from build123d import *

# Parameters (mm, degrees)
F0_R     = 4.665
F1_DEPTH = 6


with BuildPart() as f1:
    # F0 (on Front) → F1 (new body)
    with BuildSketch(Plane.XZ):
        with BuildLine():
            Line((186.500065, 187), (13.500065, 187))
            Line((13.500065, 187), (13.500065, 161.75))
            Line((13.500065, 161.75), (19.200065, 161.75))
            ThreePointArc((19.200065, 161.75), (19.412197, 161.837868), (19.500065, 162.05))
            Line((19.500065, 162.05), (19.500065, 162.8))
            ThreePointArc((19.500065, 162.8), (19.358643, 163.141421), (19.700065, 163))
            Line((19.700065, 163), (21.800065, 163))
            ThreePointArc((21.800065, 163), (22.141486, 163.141421), (22.000065, 162.8))
            Line((22.000065, 162.8), (22.000065, 162.05))
            ThreePointArc((22.000065, 162.05), (22.087933, 161.837868), (22.300065, 161.75))
            Line((22.300065, 161.75), (24.000065, 161.75))
            Line((24.000065, 161.75), (24.000065, 158.75))
            Line((24.000065, 158.75), (22.300065, 158.75))
            ThreePointArc((22.300065, 158.75), (22.087933, 158.662132), (22.000065, 158.45))
            Line((22.000065, 158.45), (22.000065, 157.7))
            ThreePointArc((22.000065, 157.7), (22.141486, 157.358579), (21.800065, 157.5))
            Line((21.800065, 157.5), (19.700065, 157.5))
            ThreePointArc((19.700065, 157.5), (19.358643, 157.358579), (19.500065, 157.7))
            Line((19.500065, 157.7), (19.500065, 158.45))
            ThreePointArc((19.500065, 158.45), (19.412197, 158.662132), (19.200065, 158.75))
            Line((19.200065, 158.75), (13.500065, 158.75))
            Line((13.500065, 158.75), (13.500065, 133.6))
            Line((13.500065, 133.6), (7.500065, 133.6))
            Line((7.500065, 133.6), (7.500065, 133.5))
            Line((7.500065, 133.5), (7.500065, 53.5))
            Line((7.500065, 53.5), (7.500065, 53.4))
            Line((7.500065, 53.4), (13.500109, 53.4))
            Line((13.500109, 53.4), (13.500072, 20.339))
            Line((13.500072, 20.339), (19.200072, 20.339))
            ThreePointArc((19.200072, 20.339), (19.412204, 20.426868), (19.500072, 20.639))
            Line((19.500072, 20.639), (19.500072, 21.389))
            ThreePointArc((19.500072, 21.389), (19.35865, 21.730421), (19.700072, 21.589))
            Line((19.700072, 21.589), (21.800072, 21.589))
            ThreePointArc((21.800072, 21.589), (22.141493, 21.730421), (22.000072, 21.389))
            Line((22.000072, 21.389), (22.000072, 20.639))
            ThreePointArc((22.000072, 20.639), (22.08794, 20.426868), (22.300072, 20.339))
            Line((22.300072, 20.339), (24.000068, 20.339))
            Line((24.000068, 20.339), (24.000068, 17.339))
            Line((24.000068, 17.339), (22.300068, 17.339))
            ThreePointArc((22.300068, 17.339), (22.087936, 17.251132), (22.000068, 17.039))
            Line((22.000068, 17.039), (22.000068, 16.289))
            ThreePointArc((22.000068, 16.289), (22.14149, 15.947579), (21.800068, 16.089))
            Line((21.800068, 16.089), (19.700068, 16.089))
            ThreePointArc((19.700068, 16.089), (19.358647, 15.947579), (19.500068, 16.289))
            Line((19.500068, 16.289), (19.500068, 17.039))
            ThreePointArc((19.500068, 17.039), (19.4122, 17.251132), (19.200068, 17.339))
            Line((19.200068, 17.339), (13.500068, 17.339))
            Line((13.500068, 17.339), (13.500031, -15.822))
            Line((13.500031, -15.822), (74.000065, -15.822))
            Line((74.000065, -15.822), (74.000065, 0))
            Line((74.000065, 0), (74.000065, 35))
            Line((74.000065, 35), (126.000065, 35))
            Line((126.000065, 35), (126.000065, 0))
            Line((126.000065, 0), (126.000065, -15.822))
            Line((126.000065, -15.822), (186.500098, -15.822))
            Line((186.500098, -15.822), (186.500061, 17.339))
            Line((186.500061, 17.339), (180.800061, 17.339))
            ThreePointArc((180.800061, 17.339), (180.587929, 17.251132), (180.500061, 17.039))
            Line((180.500061, 17.039), (180.500061, 16.289))
            ThreePointArc((180.500061, 16.289), (180.641482, 15.947579), (180.300061, 16.089))
            Line((180.300061, 16.089), (178.200058, 16.089))
            ThreePointArc((178.200058, 16.089), (177.858636, 15.947579), (178.000058, 16.289))
            Line((178.000058, 16.289), (178.000058, 17.039))
            ThreePointArc((178.000058, 17.039), (177.91219, 17.251132), (177.700058, 17.339))
            Line((177.700058, 17.339), (176.000058, 17.339))
            Line((176.000058, 17.339), (176.000058, 20.339))
            Line((176.000058, 20.339), (177.700058, 20.339))
            ThreePointArc((177.700058, 20.339), (177.91219, 20.426868), (178.000058, 20.639))
            Line((178.000058, 20.639), (178.000058, 21.389))
            ThreePointArc((178.000058, 21.389), (177.858636, 21.730421), (178.200058, 21.589))
            Line((178.200058, 21.589), (180.300058, 21.589))
            ThreePointArc((180.300058, 21.589), (180.641479, 21.730421), (180.500058, 21.389))
            Line((180.500058, 21.389), (180.500058, 20.639))
            ThreePointArc((180.500058, 20.639), (180.587926, 20.426868), (180.800058, 20.339))
            Line((180.800058, 20.339), (186.500058, 20.339))
            Line((186.500058, 20.339), (186.500021, 53.4))
            Line((186.500021, 53.4), (192.500065, 53.4))
            Line((192.500065, 53.4), (192.500065, 53.5))
            Line((192.500065, 53.5), (192.500065, 133.5))
            Line((192.500065, 133.5), (192.500065, 133.6))
            Line((192.500065, 133.6), (186.500065, 133.6))
            Line((186.500065, 133.6), (186.500065, 158.75))
            Line((186.500065, 158.75), (180.800058, 158.75))
            ThreePointArc((180.800058, 158.75), (180.587926, 158.662132), (180.500058, 158.45))
            Line((180.500058, 158.45), (180.500058, 157.7))
            ThreePointArc((180.500058, 157.7), (180.641479, 157.358579), (180.300058, 157.5))
            Line((180.300058, 157.5), (178.200058, 157.5))
            ThreePointArc((178.200058, 157.5), (177.858636, 157.358579), (178.000058, 157.7))
            Line((178.000058, 157.7), (178.000058, 158.45))
            ThreePointArc((178.000058, 158.45), (177.91219, 158.662132), (177.700058, 158.75))
            Line((177.700058, 158.75), (176.000058, 158.75))
            Line((176.000058, 158.75), (176.000058, 161.75))
            Line((176.000058, 161.75), (177.700058, 161.75))
            ThreePointArc((177.700058, 161.75), (177.91219, 161.837868), (178.000058, 162.05))
            Line((178.000058, 162.05), (178.000058, 162.8))
            ThreePointArc((178.000058, 162.8), (177.858636, 163.141421), (178.200058, 163))
            Line((178.200058, 163), (180.300065, 163))
            ThreePointArc((180.300065, 163), (180.641486, 163.141421), (180.500065, 162.8))
            Line((180.500065, 162.8), (180.500065, 162.05))
            ThreePointArc((180.500065, 162.05), (180.587933, 161.837868), (180.800065, 161.75))
            Line((180.800065, 161.75), (186.500065, 161.75))
            Line((186.500065, 161.75), (186.500065, 187))
        make_face()
        with BuildLine():
            Line((66.500065, -11.322), (66.500065, -8.322))
            ThreePointArc((66.500065, -8.322), (68.000065, -6.822), (69.500065, -8.322))
            Line((69.500065, -8.322), (69.500065, -11.322))
            ThreePointArc((69.500065, -11.322), (68.000065, -12.822), (66.500065, -11.322))
        make_face(mode=Mode.SUBTRACT)
        Polygon((28.62622, 48.081567), (28.837529, 48.534721), (65.08984, 31.629991), (64.878531, 31.176837), align=None, mode=Mode.SUBTRACT)
        with BuildLine():
            Line((130.500065, -11.322), (130.500065, -8.322))
            ThreePointArc((130.500065, -8.322), (132.000065, -6.822), (133.500065, -8.322))
            Line((133.500065, -8.322), (133.500065, -11.322))
            ThreePointArc((133.500065, -11.322), (132.000065, -12.822), (130.500065, -11.322))
        make_face(mode=Mode.SUBTRACT)
        with Locations((100.000065, 44.5)):
            Circle(F0_R, mode=Mode.SUBTRACT)
        Polygon((135.121598, 31.176837), (134.910289, 31.629991), (171.1626, 48.534721), (171.37391, 48.081567), align=None, mode=Mode.SUBTRACT)
        with BuildLine():
            ThreePointArc((9.000065, 93.75), (10.500065, 95.25), (12.000065, 93.75))
            Line((12.000065, 93.75), (12.000065, 93.25))
            ThreePointArc((12.000065, 93.25), (10.500065, 91.75), (9.000065, 93.25))
            Line((9.000065, 93.25), (9.000065, 93.75))
        make_face(mode=Mode.SUBTRACT)
        with BuildLine():
            Line((191.000064, 93.75), (191.000064, 93.25))
            ThreePointArc((191.000064, 93.25), (189.500064, 91.75), (188.000064, 93.25))
            Line((188.000064, 93.25), (188.000064, 93.75))
            ThreePointArc((188.000064, 93.75), (189.500064, 95.25), (191.000064, 93.75))
        make_face(mode=Mode.SUBTRACT)
    extrude(amount=F1_DEPTH)


solid = f1.part
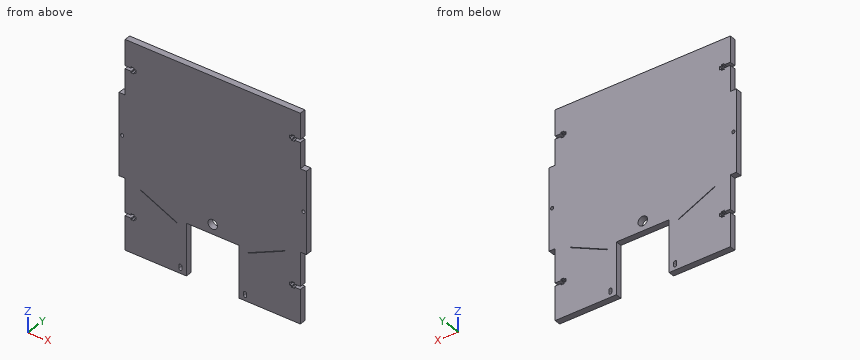
Work out the finished part from the listing and answer in its coordinate system (mm). Round coordinates to 2 decimals unless told otherwise and drop trailing zeros. Loops run counter-clockwise (first coordinate to the right, second up) from the corner with the lowest first, then second, coordinate; pieces in that order, holes last. Notation, with made-up numbers: (-9.75, 70.5) - (1.25, 70.5) arc R3 ccw to (1.25, 75.5) - close; hole circle Ø9 at (-7, -29). An arc over 180 degrees is marked (long way). One line per item, written item: value.
Q1. Find section A-A on z = 44.5. Give the vertices of the cut face in (x, y), and give its area (3 significant figures).
Check values:
outline: (13.5, -6) - (36.31, -6) - (36.31, 0) - (13.5, 0) - close; (37.49, -6) - (95.34, -6) - (95.34, 0) - (37.49, 0) - close; (104.67, -6) - (162.51, -6) - (162.51, 0) - (104.67, 0) - close; (163.69, -6) - (186.5, -6) - (186.5, 0) - (163.69, 0) - close
area: 968 mm2
Q2. Find section C-C on x = 107.5. Give the vertices of the cut face in (y, z).
Check values:
outline: (-6, 35) - (0, 35) - (0, 187) - (-6, 187) - close
Q3. Straight lines are drawn through the part: probe 1 along Z at (x, y) = (185, -5.7); probe 2 along X at (y, z) = (-3.6, 15.5); probe 3 along Z at (x, y) = (100, -2.9) (3 decimals). For each, find the intervals that lie inside material, in ascending order.
Check values:
probe 1: -15.82 to 17.34, 20.34 to 158.75, 161.75 to 187
probe 2: 13.5 to 74, 126 to 186.5
probe 3: 35 to 39.835, 49.165 to 187
Q4. Find section B-B on y = -2. State how many separate pieces and enclosed holes the cut face has, and give its area (3 significant figures).
Check values:
separate pieces: 1
enclosed holes: 7
area: 33,100 mm2
Q5. Each of these flat-tipped pins is pushed along its axis until it touches: pin 1 Ø3.5 at (y, z) = (-2.5, 19.5) entering from +X; pin 2 Ø3 at (x, z) = (107.5, 49.5) entering from +Y. Where does it stop, or does it pass through?
Check values:
pin 1: x = 186.5
pin 2: y = 0
